Part model, mm, in its own coordinate system. A direction names the side the tool comes from. Coordinates: 2 decimals unless noted, no trailing zeros. Write each loop counter-clockwise with the first axis right and the second up, starting at its lowest first coordinate (ties: lowest second). Pieces come first, ordered by that corner, then holes. Notation, with made-up numbers: (-26, 29) -> (19, 29) arc R10 ccw to (19, 36) -> close; hole circle Ø8 at (-34, -16.5). An arc over 180 degrees is marked (long way). One line per question, with ' | ' between items. Start each with the question number.
Item 1: Pin check, flat tip, straight feed: pin 1 (1 mm diameter, centred on x = 111, z = 6.5, fed in from +Y). Stop position of the tip, or through.
Item 2: Saw through at D-D (x = 316). List the corners of the cut face in (y, z), and give its area (3 significant figures).
Item 3: Saw through at B-B (z = 5.5). List the corners of the cut face in (x, y).
Item 4: Saw through at A-A (y = 127.5). List the corners of the cut face in (x, z), and give its area (3 significant figures).
Item 5: 3-axis set-ups, long thin cutter, end or side, ignore diameter. For faces 1 (the cylindrical face through (435.774, 138.836, 3.944)), 2 (the flat face through (222, 71, 8)): which of +Z, -Z, +X, -X, +Y, -Y reach the whole face in a straight line?
Item 6: Probe probe 1 along Y at (x, z) = (335.5, 0.5); probe 2 along X at (y, z) = (7.5, 5.5); probe 3 along Y at (x, z) = (306.5, 7.75). List the from-to ranges inside material, lowest first. Write a range as [from, to].
Item 7: Saw through at C-C (x = 57). List the corners of the cut face in (y, z), and give its area (3 significant figures).
Item 8: Two-plate mould, pull along X, no slides. Class faces 3 (the cylindrical face through (14.35, 138.77, 3.94)), 4 (the cylindrical face through (446.99, 2.85, 3.94)), 5 (the flat face through (222, 71, 0)), 6 (the flat face through (0, 73, 4)): pulls with the +X half, pulls with the -X half, needs draft (parallel to the pull), parting line crosses it, or undercut.
from build123d import *

# Parameters (mm, degrees)
ESQUISSE1_W                  = 450
ESQUISSE1_H                  = 140
BOSS_EXTRU_1_DEPTH           = 8
ENL_V_MAT_EXTRU_1_DEPTH      = 472.342762753
ENL_V_MAT_EXTRU_1_DEPTH_BACK = 472.342762753
ESQUISSE2_R                  = 35.45
CONG_1_R                     = 10
CONG_2_R                     = 3


with BuildPart() as part:
    # Esquisse1 → Boss.-Extru.1 (new body)
    with BuildSketch(Plane.XY):
        with Locations((225, 70)):
            Rectangle(ESQUISSE1_W, ESQUISSE1_H)
    extrude(amount=BOSS_EXTRU_1_DEPTH)

    # Esquisse2 → Enlèv. mat.-Extru.1 (cut, two sides: drawn at the far end of the back side and taken through both)
    with BuildSketch(Plane.XY.offset(8).offset(-ENL_V_MAT_EXTRU_1_DEPTH_BACK)):
        with Locations((189.5, 155)):
            Circle(ESQUISSE2_R)
        with Locations((118.5, 155)):
            Circle(ESQUISSE2_R)
        with Locations((47.5, 155)):
            Circle(ESQUISSE2_R)
        with Locations((402.5, 155)):
            Circle(ESQUISSE2_R)
        with Locations((331.5, 155)):
            Circle(ESQUISSE2_R)
        with Locations((260.5, 155)):
            Circle(ESQUISSE2_R)
    extrude(amount=ENL_V_MAT_EXTRU_1_DEPTH + ENL_V_MAT_EXTRU_1_DEPTH_BACK, mode=Mode.SUBTRACT)

    # Congé1
    # the kernel refuses this fillet: 10 mm, written as the material it takes off along each edge
    with BuildSketch(Plane(origin=(221.620126089, 140, -14.591152386), x_dir=(-0.4878841610391912, -0.87290838316921, 0), z_dir=(0, 0, 1)), Plane(origin=(150.620126089, 140, -14.591152386), x_dir=(-0.4878841610391912, -0.87290838316921, 0), z_dir=(0, 0, 1)), Plane(origin=(79.620126089, 140, -14.591152386), x_dir=(-0.4878841610391912, -0.87290838316921, 0), z_dir=(0, 0, 1)), Plane(origin=(363.620126089, 140, -14.591152386), x_dir=(-0.48788416103919546, -0.8729083831692078, 0), z_dir=(0, 0, 1)), Plane(origin=(292.620126089, 140, -14.591152386), x_dir=(-0.48788416103919546, -0.8729083831692078, 0), z_dir=(0, 0, 1))) as cong_1_piece_1:
        with BuildLine():
            CenterArc((5.881566976, 9.973537305), CONG_1_R, 209.201608238, 56.629213342)
            Line((-2.847516856, 5.094695695), (0, 0))
            ThreePointArc((0, 0), (2.577275022, 0.093810253), (5.154550044, 0))
        make_face()
    extrude(amount=37.182304771, mode=Mode.SUBTRACT)
    with BuildSketch(Plane(origin=(157.379873911, 140, -14.591152386), x_dir=(-1, 0, 0), z_dir=(0, 0, 1)), Plane(origin=(86.379873911, 140, -14.591152386), x_dir=(-1, 0, 0), z_dir=(0, 0, 1)), Plane(origin=(15.379873911, 140, -14.591152386), x_dir=(-1, 0, 0), z_dir=(0, 0, 1)), Plane(origin=(370.379873911, 140, -14.591152386), x_dir=(-1, 0, 0), z_dir=(0, 0, 1)), Plane(origin=(299.379873911, 140, -14.591152386), x_dir=(-1, 0, 0), z_dir=(0, 0, 1)), Plane(origin=(228.379873911, 140, -14.591152386), x_dir=(-1, 0, 0), z_dir=(0, 0, 1))) as cong_1_piece_2:
        with BuildLine():
            CenterArc((5.836460954, 10), CONG_1_R, 213.370786658, 56.629213342)
            ThreePointArc((-2.514823324, 4.499449945), (-1.175523906, 2.295493509), (0, 0))
            Line((0, 0), (5.836460954, 0))
        make_face()
    extrude(amount=37.182304771, mode=Mode.SUBTRACT)
    with BuildSketch(Plane(origin=(434.620126089, 140, -14.591152386), x_dir=(1, 0, 0), z_dir=(0, 0, 1))) as cong_1_piece_3:
        with BuildLine():
            CenterArc((5.836460954, -10), CONG_1_R, 90, 56.629213342)
            ThreePointArc((-2.514823324, -4.499449945), (-1.175523906, -2.295493509), (0, 0))
            Line((0, 0), (5.836460954, 0))
        make_face()
    extrude(amount=37.182304771, mode=Mode.SUBTRACT)
    with BuildSketch(Plane(origin=(450, 0, -25), x_dir=(-1, 0, 0), z_dir=(0, 0, 1))) as cong_1_piece_4:
        with BuildLine():
            CenterArc((CONG_1_R, -CONG_1_R), CONG_1_R, 90, 90)
            Line((0, -CONG_1_R), (0, 0))
            Line((0, 0), (CONG_1_R, 0))
        make_face()
    extrude(amount=58, mode=Mode.SUBTRACT)
    with BuildSketch(Plane(origin=(0, 0, -25), x_dir=(1, 0, 0), z_dir=(0, 0, 1))) as cong_1_piece_5:
        with BuildLine():
            CenterArc((CONG_1_R, CONG_1_R), CONG_1_R, 180, 90)
            Line((0, CONG_1_R), (0, 0))
            Line((0, 0), (CONG_1_R, 0))
        make_face()
    extrude(amount=58, mode=Mode.SUBTRACT)

    # Congé2
    cong_2_edges = [part.edges().sort_by_distance(p)[0] for p in [
        (0, 140, 4),
        (450, 140, 4),
    ]]
    fillet(cong_2_edges, radius=CONG_2_R)


solid = part.part
From the geometry:
1) pin 1: y = 120.46
2) outline: (0, 0) -> (123.12, 0) -> (123.12, 8) -> (0, 8) -> close | area: 985 mm2
3) outline: (0, 10) arc R10 ccw to (10, 0) -> (440, 0) arc R10 ccw to (450, 10) -> (450, 137) arc R3 ccw to (447, 140) -> (440.46, 140) arc R10 ccw to (432.11, 135.5) arc R35.45 cw to (372.89, 135.5) arc R10 ccw to (367, 139.69) arc R10 ccw to (361.11, 135.5) arc R35.45 cw to (301.89, 135.5) arc R10 ccw to (296, 139.69) arc R10 ccw to (290.11, 135.5) arc R35.45 cw to (230.89, 135.5) arc R10 ccw to (225, 139.69) arc R10 ccw to (219.11, 135.5) arc R35.45 cw to (159.89, 135.5) arc R10 ccw to (154, 139.69) arc R10 ccw to (148.11, 135.5) arc R35.45 cw to (88.89, 135.5) arc R10 ccw to (83, 139.69) arc R10 ccw to (77.11, 135.5) arc R35.45 cw to (17.89, 135.5) arc R10 ccw to (9.54, 140) -> (3, 140) arc R3 ccw to (0, 137) -> close
4) outline: (0, 0) -> (25.13, 0) -> (25.13, 8) -> (0, 8) -> close; (69.87, 0) -> (96.13, 0) -> (96.13, 8) -> (69.87, 8) -> close; (140.87, 0) -> (167.13, 0) -> (167.13, 8) -> (140.87, 8) -> close; (211.87, 0) -> (238.13, 0) -> (238.13, 8) -> (211.87, 8) -> close; (282.87, 0) -> (309.13, 0) -> (309.13, 8) -> (282.87, 8) -> close; (353.87, 0) -> (380.13, 0) -> (380.13, 8) -> (353.87, 8) -> close; (424.87, 0) -> (450, 0) -> (450, 8) -> (424.87, 8) -> close | area: 1,450 mm2
5) face 1: +Z, -Z, +Y | face 2: +Z, +X, -X, +Y, -Y
6) probe 1: [0, 119.78] | probe 2: [0.32, 449.68] | probe 3: [0, 129.87]
7) outline: (0, 0) -> (120.85, 0) -> (120.85, 8) -> (0, 8) -> close | area: 967 mm2
8) face 3: undercut | face 4: pulls with the +X half | face 5: needs draft | face 6: pulls with the -X half
